Answer from the drawing. Dimensions are ordinates in mm from the lowest x, y and z of the part. A direction names the side the tool comes from. Coordinates: 2 decimals unless noted, no trailing zeros. Order: outer loops, then holes, each group sorted by start corner. A loop starts at its lowest first (then second) coordinate and runs counter-clockwise, first axis right, second up.
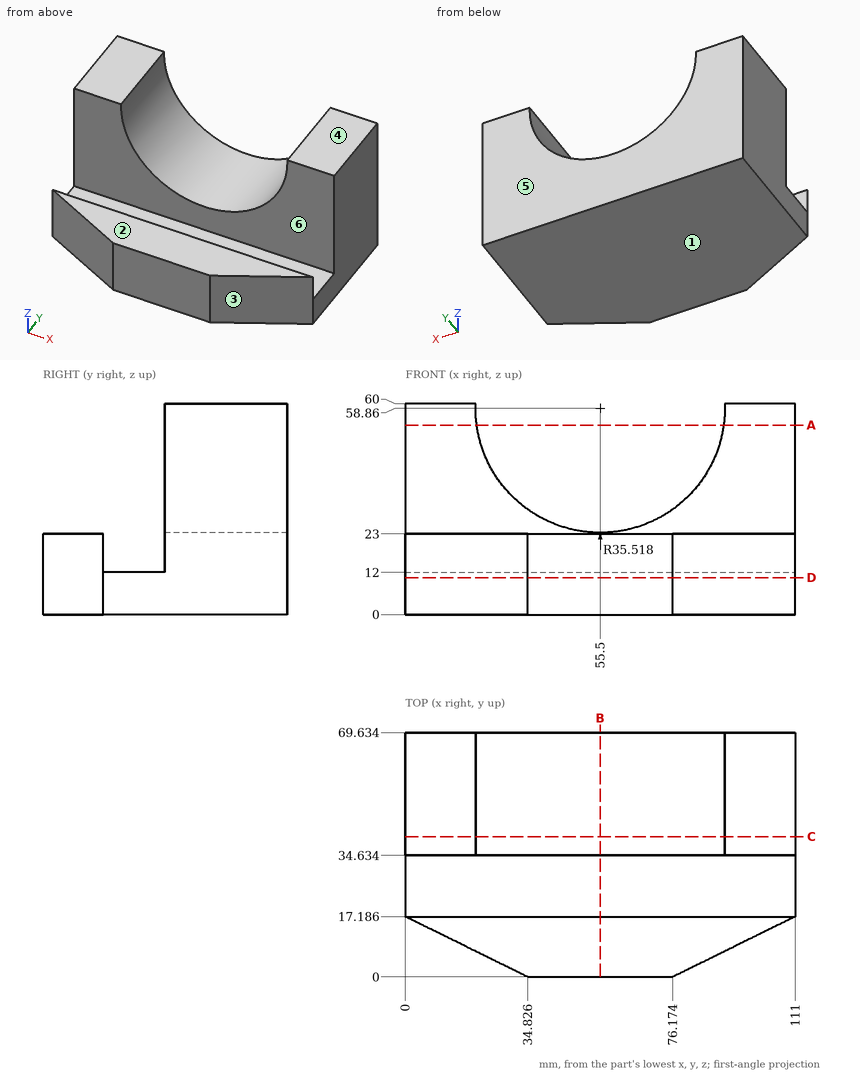
1. The part is cut by section C-C (y = 40). Determine the outline of the cut face in (x, z), plus the area to 3 significant figures.
2. The mould has two halves that part along Y. Classify the marked faces 3, 4, 5 and 6: released by +Y, released by -Y, zero draft, split by the parting line, or undercut.
3. The part is cut by section B-B (x = 55.5). Determine the outline of the cut face in (y, z) (1 decimal).
4. For the marked faces 1 and 2, determine the directions among +Z, -Z, +X, -X, +Y, -Y from which every point of the face is accessible in a straight line to the end or side of a thin tool.
5. The part is cut by section A-A (z = 54). Determine the outline of the cut face in (x, y), plus the area to 3 significant figures.
6. The part is cut by section D-D (z = 10.5). Determine the outline of the cut face in (x, y) (1 decimal), plus the area to 3 significant figures.
7. Flat-ended cylindrical pins translate along their axes: pin 1 (8.5 mm diameter, centred on x = 49.5, y = 26.5, fed in from +Z); pin 2 (1.5 mm diameter, centred on x = 16.5, z = 11, fed in from -Y); pin 3 (8.5 mm diameter, centred on x = 73.5, y = 7, fed in from +Z). Find the tip coordinate at first contact, or state that the pin passes through.
8. Consider probe 1 along Z at (x, y) = (39, 28.5); probe 2 along X at (y, z) = (43, 57); probe 3 along X at (y, z) = (47.5, 51.5). Determine where each line is inside the solid, lowest interval first.
Worked out:
1. outline: (0, 0) - (111, 0) - (111, 60) - (91, 60) arc R35.52 cw (long way) to (20, 60) - (0, 60) - close
1. area: 4,600 mm2
2. face 3: released by -Y
2. face 4: zero draft
2. face 5: released by +Y
2. face 6: undercut
3. outline: (0, 0) - (69.6, 0) - (69.6, 23.3) - (34.6, 23.3) - (34.6, 12) - (17.2, 12) - (17.2, 23) - (0, 23) - close
4. face 1: -Z, +X, -X, +Y, -Y
4. face 2: +Z, +X, -X, -Y
5. outline: (0, 34.63) - (20.32, 34.63) - (20.32, 69.63) - (0, 69.63) - close; (90.68, 34.63) - (111, 34.63) - (111, 69.63) - (90.68, 69.63) - close
5. area: 1,420 mm2
6. outline: (0, 17.2) - (34.8, 0) - (76.2, 0) - (111, 17.2) - (111, 69.6) - (0, 69.6) - close
6. area: 7,130 mm2
7. pin 1: stops at z = 12
7. pin 2: stops at y = 8.67
7. pin 3: stops at z = 23
8. probe 1: z = 0 to 12
8. probe 2: x = 0 to 20.03, 90.97 to 111
8. probe 3: x = 0 to 20.75, 90.25 to 111
